```python
from build123d import *

# Parameters (mm, degrees)
SKETCH1_W           = 70
SKETCH1_H           = 70
BOSS_EXTRUDE1_DEPTH = 13.5
SKETCH5_R           = 1.55
FANS_COLUMN_DEPTH   = 14
SKETCH6_R           = 17.5
CUT_EXTRUDE2_DEPTH  = 15
FILLET1_R           = 1.5
SKETCH7_R           = 2.5
BOSS_EXTRUDE4_DEPTH = 31.75
SKETCH8_W           = 3
SKETCH8_H           = 4
CUT_EXTRUDE3_DEPTH  = 22
BOSS_EXTRUDE5_DEPTH = 10
SKETCH10_W          = 30
SKETCH10_H          = 10.5
CUT_EXTRUDE4_DEPTH  = 95.723611148
SKETCH11_W          = 30
SKETCH11_H          = 10
CUT_EXTRUDE5_DEPTH  = 99.349186657


with BuildPart() as part:
    # Sketch1 → Boss-Extrude1 (new body)
    with BuildSketch(Plane(origin=(0, 0, 0), x_dir=(1, 0, 0), z_dir=(0, 1, 0))):
        Rectangle(SKETCH1_W, SKETCH1_H)
    extrude(amount=BOSS_EXTRUDE1_DEPTH)

    # Sketch5 → Fans_Column (add)
    with BuildSketch(Plane(origin=(0, 13.5, 0), x_dir=(1, 0, 0), z_dir=(0, 1, 0))):
        with Locations(Location((-16.35, 16.35, 0), (0, 0, 90))):
            Circle(SKETCH5_R)
        with Locations(Location((16.35, 16.35, 0), (0, 0, 90))):
            Circle(SKETCH5_R)
        with Locations(Location((16.35, -16.35, 0), (0, 0, 90))):
            Circle(SKETCH5_R)
        with Locations(Location((-16.35, -16.35, 0), (0, 0, 90))):
            Circle(SKETCH5_R)
    extrude(amount=FANS_COLUMN_DEPTH)

    # Sketch6 → Cut-Extrude2 (cut)
    with BuildSketch(Plane(origin=(0, 13.5, 0), x_dir=(1, 0, 0), z_dir=(0, 1, 0))):
        with Locations(Location((0, 0, 0), (0, 0, 270))):
            Circle(SKETCH6_R)
    extrude(amount=-CUT_EXTRUDE2_DEPTH, mode=Mode.SUBTRACT)

    # Fillet1
    fillet1_edges = [part.edges().sort_by_distance(p)[0] for p in [
        (0, 13.5, -17.5),
    ]]
    fillet(fillet1_edges, radius=FILLET1_R)

    # Sketch7 → Boss-Extrude4 (add)
    with BuildSketch(Plane(origin=(0, 13.5, 0), x_dir=(1, 0, 0), z_dir=(0, 1, 0))):
        with Locations(Location((-31.5, -31.5, 0), (0, 0, 270))):
            Circle(SKETCH7_R)
        with Locations(Location((-31.5, 31.5, 0), (0, 0, 90))):
            Circle(SKETCH7_R)
        with Locations(Location((31.5, 31.5, 0), (0, 0, 270))):
            Circle(SKETCH7_R)
        with Locations(Location((31.5, -31.5, 0), (0, 0, 90))):
            Circle(SKETCH7_R)
    extrude(amount=BOSS_EXTRUDE4_DEPTH)

    # Sketch8 → Cut-Extrude3 (cut)
    with BuildSketch(Plane.XY.offset(35)):
        with Locations((-9.518750433, 11.5)):
            Rectangle(SKETCH8_W, SKETCH8_H)
    extrude(amount=-CUT_EXTRUDE3_DEPTH, mode=Mode.SUBTRACT)

    # Sketch9 → Boss-Extrude5 (add)
    with BuildSketch(Plane.XY.offset(35)):
        Polygon((-8.018750433, 9.5), (-11.018750433, 9.5), (-11.018750433, 13.5), (-35, 13.5), (-35, 0), (35, 0), (35, 13.5), (-8.018750433, 13.5), align=None)
    extrude(amount=BOSS_EXTRUDE5_DEPTH)

    # Sketch10 → Cut-Extrude4 (cut, through all)
    with BuildSketch(Plane.ZY.offset(35)):
        with Locations((0.031213212, 5.25)):
            Rectangle(SKETCH10_W, SKETCH10_H)
    extrude(amount=-CUT_EXTRUDE4_DEPTH, mode=Mode.SUBTRACT)

    # Sketch11 → Cut-Extrude5 (cut, through all)
    with BuildSketch(Plane(origin=(0, 0, -35), x_dir=(-1, 0, 0), z_dir=(0, 0, -1))):
        with Locations((0, 5)):
            Rectangle(SKETCH11_W, SKETCH11_H)
    extrude(amount=-CUT_EXTRUDE5_DEPTH, mode=Mode.SUBTRACT)


solid = part.part
```
Design review of the part built by this model. Coordinates are the model's own, in mm. A direction names the side the tool comes from. Give positions to 0.01 mm unless a question says otherwise; leave off trailing zeros. Loops run counter-clockwise (first coordinate to the right, second up) from the corner with the lowest first, then second, coordinate; pieces in that order, holes last. Notation, with made-up numbers: (26, 80) -> (50, 80) arc R12 ccw to (50, 98) -> close; hole circle Ø6 at (56, -39). An arc over 180 degrees is marked (long way). Write each question's results on one line, items separated by ' | '.
Q1. The part is to be moulded in two halves that separate along Z. For faces 1 (the face through (33.19, 29.15, -33.34)), 2 (the face through (-23, 7, 45)), 3 (the face through (25, 5, 15.031)), 4 (the face through (32, 45.25, -32)), say which applies: +Z half, -Z half, draft (parallel to the pull), parting line (faces both ways), or undercut.
Reply:
face 1: undercut | face 2: +Z half | face 3: undercut | face 4: draft
Q2. Wall thickness on L1, parallel to Z at x = 0, y = 11; L2, parallel to X at y = 11, z = 0; L3, parallel to X at y = 12, z = 20.5: over which ranges is each line inside the solid? List them lowest first.
Reply:
L1: z = -35 to -17.5, 17.5 to 45 | L2: x = -35 to -17.5, 17.5 to 35 | L3: x = -35 to -11.02, -8.02 to 35
Q3. Take a section at B-B, the plane x = 0. Write out the cut boundary in (y, z).
Reply:
outline: (10, -35) -> (13.5, -35) -> (13.5, -19) arc R1.5 ccw to (12, -17.5) -> (10, -17.5) -> close; (10, 17.5) -> (12, 17.5) arc R1.5 ccw to (13.5, 19) -> (13.5, 45) -> (10, 45) -> close
Q4. Machinability: for faces 5 (the face through (-16.816, 20.402, 14.872)), 6 (the face through (-32, 45.25, -31)), 7 (the face through (25, 0, 30)), 8 (the face through (-25, 10.5, 0)), 9 (the face through (-13, 10, 30)), which of the approach directions +Z, -Z, +X, -X, +Y, -Y give a long, thin tool a straight path to every point of the face, cutting with its end or side? Answer none if there is none.
Reply:
face 5: +Y | face 6: +Z, -Z, +X, -X, +Y | face 7: +Z, -Z, +X, -X, -Y | face 8: +X, -X, -Y | face 9: +Z, -Z, -Y
Q5. For pin 1 Ø1.5 at (x, z) = (2.5, -24) entering from +Y; pin 2 Ø3 at (x, z) = (-12.5, 33.5) entering from -Y; pin 3 Ø8 at (x, y) = (14.5, 23) entering from -Z, all flat-tipped, find the tip position at first contact; note any pin that passes through.
Reply:
pin 1: stops at y = 13.5 | pin 2: stops at y = 10 | pin 3: stops at z = -17.9
Q6. Take a section at D-D, the plane x = 22. Write out the cut boundary in (y, z), plus the area to 3 significant figures.
Reply:
outline: (0, -35) -> (13.5, -35) -> (13.5, 45) -> (0, 45) -> (0, 15.03) -> (10.5, 15.03) -> (10.5, -14.97) -> (0, -14.97) -> close | area: 765 mm²
Q7. Take a section at C-C, the plane y = 8.5. Write out the cut boundary in (x, z).
Reply:
outline: (-35, -35) -> (-15, -35) -> (-15, -14.97) -> (-35, -14.97) -> close; (-35, 15.03) -> (-15, 15.03) -> (-15, 45) -> (-35, 45) -> close; (15, -35) -> (35, -35) -> (35, -14.97) -> (15, -14.97) -> close; (15, 15.03) -> (35, 15.03) -> (35, 45) -> (15, 45) -> close
Q8. Take a section at A-A, the plane y = 24. Write out the cut boundary in (x, z), plus the area to 3 significant figures.
Reply:
outline: circle Ø5 at (-31.5, -31.5); circle Ø5 at (-31.5, 31.5); circle Ø3.1 at (-16.35, -16.35); circle Ø3.1 at (-16.35, 16.35); circle Ø3.1 at (16.35, -16.35); circle Ø3.1 at (16.35, 16.35); circle Ø5 at (31.5, -31.5); circle Ø5 at (31.5, 31.5) | area: 109 mm²
